Part model, mm, in its own coordinate system. Face numbers are marked on the shaded views. A direction names the side the tool comes from. Round coordinates to 2 decimals unless told otherwise and drop trailing zeros. Loops run counter-clockwise (first coordinate to the right, second up) from the corner with the lowest first, then second, coordinate; pieces in that order, holes last.
(1) Tool access for the marked faces 1, 2 and 3: list every direction of +Z, -Z, +X, -X, +Y, -Y with a clear straight run to the whole face (end or side of a thin tool).
(2) Cut at A-A on x = 21.75. List the corners of the cut face in (y, z).
(3) Probe probe 1 along Z at (x, y) = (20.75, 9.25); probe 2 along Z at (x, y) = (13.5, 10.25); probe 3 along Z at (x, y) = (13.75, 10.75). List the from-to ranges inside material, lowest first.
(4) Flat gauge pins, fed straight in: pin 1 (1 mm diameter, centred on x = 14, z = 4, fed in from +Y); pin 2 (1 mm diameter, centred on y = 14, z = 8, fed in from -X); pin 3 (0.6 mm diameter, centred on x = 17, y = 11.5, fed in from -Z); pin 4 (2 mm diameter, centred on x = 17, y = 12, fed in from +Z). Where does each tip first touch, or does it go through?
from build123d import *

# Parameters (mm, degrees)
P_IDAT_VYSUNUT_M2_DEPTH  = 15
SKICA3_W                 = 28.958839484
SKICA3_H                 = 34.368053108
ODEBRAT_VYSUNUT_M2_DEPTH = 19.470465231
ZAOBLIT7_R               = 1
ZAOBLIT8_SIZE            = 5
ZAOBLIT8_SIZE_2          = 1


# Read off the part's stored shape, not the designer's step: Přidat vysunutím2
with BuildPart() as part:
    # Skica1 → Rotovat1 (revolve)
    with BuildSketch(Plane.XY, mode=Mode.PRIVATE) as rotovat1_sk:
        with BuildLine():
            Line((-18.006318941, 12.994441011), (-18.006318941, 0))
            Line((-18.006318941, 0), (-15.006318941, 0))
            Line((-15.006318941, 0), (-15.006318941, 10.5))
            Line((-15.006318941, 10.5), (-5.006318941, 10.5))
            Line((-5.006318941, 10.5), (-5.006318941, 12.5))
            Line((-5.006318941, 12.5), (7.993681059, 12.5))
            Line((7.993681059, 12.5), (9.993681059, 12.604815559))
            Line((9.993681059, 12.604815559), (9.993681059, 14.5))
            ThreePointArc((9.993681059, 14.5), (9.70078784, 15.207106781), (8.993681059, 15.5))
            Line((8.993681059, 15.5), (-4.506318941, 15.5))
            Line((-4.506318941, 15.5), (-18.006318941, 12.994441011))
        make_face()
    revolve(rotovat1_sk.sketch.rotate(Axis((-22.002499385, 0, 0), (1, 0, 0)), 90), axis=Axis((-22.002499385, 0, 0), (1, 0, 0)))

    # Přidat vysunutím2 outline → Přidat vysunutím2 (add)
    with BuildSketch(Plane(origin=(9.993681059, 0, 0), x_dir=(0, 0, -1), z_dir=(1, 0, 0))):
        with BuildLine():
            ThreePointArc((9, 12.619429464), (0, 15.5), (-9, 12.619429464))
            Line((-9, 12.619429464), (-9, 10.677226605))
            ThreePointArc((-9, 10.677226605), (-9.838449164, 9.89820076), (-10.609715537, 9.052608394))
            Line((-10.609715537, 9.052608394), (-9.920275538, 8.474099545))
            ThreePointArc((-9.920275538, 8.474099545), (-9.473009337, 8.979756174), (-9, 9.461417722))
            Line((-9, 9.461417722), (-9, 8.752470575))
            ThreePointArc((-9, 8.752470575), (0, 12.6), (9, 8.752470575))
            Line((9, 8.752470575), (9, 9.461417722))
            ThreePointArc((9, 9.461417722), (9.473009337, 8.979756174), (9.920275538, 8.474099545))
            Line((9.920275538, 8.474099545), (10.609715537, 9.052608394))
            ThreePointArc((10.609715537, 9.052608394), (9.838449164, 9.89820076), (9, 10.677226605))
            Line((9, 10.677226605), (9, 12.619429464))
        make_face()
    extrude(amount=P_IDAT_VYSUNUT_M2_DEPTH)

    # Skica3 → Odebrat vysunutím2 (cut, symmetric)
    with BuildSketch(Plane.XY):
        with Locations((-4.485738683, -0.096675255)):
            Rectangle(SKICA3_W, SKICA3_H)
    extrude(amount=ODEBRAT_VYSUNUT_M2_DEPTH, both=True, mode=Mode.SUBTRACT)

    # Zaoblit7
    zaoblit7_edges = [part.edges().sort_by_distance(p)[0] for p in [
        (24.993681059, 15.5, 0),
    ]]
    fillet(zaoblit7_edges, radius=ZAOBLIT7_R)

    # Zaoblit8
    # an asymmetric fillet: 5, 1 mm, written as the material it takes off along each edge
    with BuildSketch(Plane(origin=(9.993681059, 1e-09, 0), x_dir=(0, 0.1441186549809942, -0.9895604141670529), z_dir=(0, -0.9895604141670529, -0.1441186549809942))) as zaoblit8_piece_1:
        with BuildLine():
            Bezier((15.499999999, ZAOBLIT8_SIZE), (15.499999999, 0), (15.499999999 - ZAOBLIT8_SIZE_2, 0), weights=[1, 0.707106781, 1])
            Line((15.499999999 - ZAOBLIT8_SIZE_2, 0), (15.499999999, 0))
            Line((15.499999999, 0), (15.499999999, ZAOBLIT8_SIZE))
        make_face()
    revolve(axis=Axis((9.993681059, 1e-09, 0), (1, 0, 0)), revolution_arc=163.427508421, mode=Mode.SUBTRACT)


solid = part.part
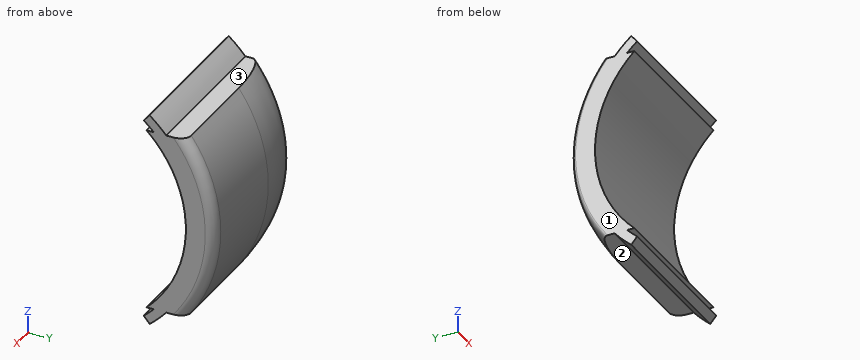
Final values:
1. face 1: +Z, -Z, -X, +Y, -Y
1. face 2: -Z, +X, -X, +Y
1. face 3: +Z, +X, -X, +Y
2. outline: (8.47, -9.92) - (9.05, -10.61) arc R13.85 ccw to (10.68, -9) - (12.62, -9) arc R15.5 ccw to (12.62, 9) - (10.68, 9) arc R13.85 ccw to (9.05, 10.61) - (8.47, 9.92) arc R12.95 cw to (9.46, 9) - (8.75, 9) arc R12.45 cw to (8.75, -9) - (9.46, -9) arc R12.95 cw to start
3. probe 1: z = -10.44 to -9.21, -9 to -8.5, 8.5 to 9, 9.21 to 10.44
3. probe 2: z = -9.48 to -7.28, 7.28 to 9.48
3. probe 3: z = -9 to -6.53, 6.53 to 9
4. pin 1: stops at y = 15.08
4. pin 2: passes through
4. pin 3: stops at z = -9
4. pin 4: stops at z = 9
